Work out the finished part from the listing and answer in its coordinate system (mm). A direction names the side the tool comes from. Coordinates: 2 decimals unless noted, no trailing zeros. Loops run counter-clockwise (first coordinate to the right, second up) from the corner with the lowest first, then second, coordinate; pieces in that order, holes last.
Autodesk Inventor part; units mm, degrees
ref_plane "YZ Plane" through (0, 0, 0) normal (1, 0, 0) x (0, 1, 0)
ref_plane "XZ Plane" through (0, 0, 0) normal (0, 1, 0) x (-1, 0, 0)
ref_plane "XY Plane" through (0, 0, 0) normal (0, 0, 1) x (1, 0, 0)
sketch "Sketch1" plane through (0, 0, 0) normal (0, 1, 0) x (-1, 0, 0)
  line L0 (0, 0) -> (14.859, 0)
  line L1 (14.859, 0) -> (14.859, -17.145)
  line L2 (14.859, -17.145) -> (0, -17.145)
  line L3 (0, -17.145) -> (0, 0)
  line L4 (0, 0) -> (0, -1.143)
  line L5 (0, -1.143) -> (-3.175, -1.143)
  line L6 (-3.175, -1.143) -> (-20.32, -1.143)
  line L7 (-20.32, -1.143) -> (-20.32, -16.002)
  line L8 (-20.32, -16.002) -> (-3.175, -16.002)
  line L9 (-3.175, -16.002) -> (-3.175, -1.143)
  line L10 (14.859, 0) -> (14.859, 3.175)
  line L11 (14.859, 3.175) -> (18.034, 3.175)
  line L12 (-20.32, -1.143) -> (-23.495, -1.143)
  line L13 (-20.32, -16.002) -> (-20.32, -19.177)
  line L14 (-20.32, -19.177) -> (-23.495, -19.177)
  line L15 (18.034, 3.175) -> (-23.495, 3.175)
  line L16 (-23.495, 3.175) -> (-23.495, -19.177)
  line L17 (-23.495, -19.177) -> (18.034, -19.177)
  line L18 (18.034, -19.177) -> (18.034, 3.175)
  dimension "d0" = 14.859
  dimension "d1" = 17.145
  dimension "d2" = 1.143
  dimension "d3" = 3.175
  dimension "d4" = 17.145
  dimension "d5" = 14.859
  dimension "d6" = 3.175
  dimension "d7" = 3.175
  dimension "d8" = 3.175
  dimension "d34" = 3.175
  dimension "d35" = 3.175
extrude "Extrusion1" add sketch "Sketch1" along normal blind 25.4 contours L3 L5 L6 L12 L16 L15 L10 L0 | L10 L11 L18 L17 L13 L8 L9 L5 L3 L2 L1 | L7 L13 L14 L16 L12
sketch "Sketch2" plane through (23.495, 0, 1.5875) normal (1, 0, 0) x (0, 0, -1)
  line L0 (17.5895, 25.4) -> (2.7305, 25.4)
  line L1 (10.16, 25.4) -> (10.16, 17.399)
  circle A0 centre (10.16, 17.399) radius 1.5875
  line L2 (10.16, 17.399) -> (10.16, 2.413)
  circle A1 centre (10.16, 2.413) radius 1.5875
  point P0 (1.5875, 0)
  dimension "d13" = 8.001
  dimension "d14" = 3.175
  dimension "d15" = 14.986
  dimension "d16" = 3.175
extrude "Extrusion2" cut sketch "Sketch2" against normal blind 9.525
sketch "Sketch3" plane through (19.05, 0, -19.177) normal (0, 0, -1) x (-1, 0, 0)
  line L0 (33.909, 0) -> (33.909, 25.4)
  line L1 (19.05, 0) -> (19.05, 25.4)
  line L2 (33.909, 25.4) -> (19.05, 25.4)
  line L3 (26.4795, 25.4) -> (26.4795, 17.399)
  circle A0 centre (26.4795, 17.399) radius 1.5875
  line L4 (26.4795, 17.399) -> (26.4795, 2.413)
  circle A1 centre (26.4795, 2.413) radius 1.5875
  dimension "d19" = 8.001
  dimension "d20" = 3.175
  dimension "d21" = 14.986
  dimension "d22" = 3.175
extrude "Extrusion3" cut sketch "Sketch3" against normal blind 9.525
move faces "Move1" translate (0, -1.5875, 0) faces at (1.8203, 0, 2.1167)
sketch "Sketch4" plane through (-18.034, 25.4, -17.4625) normal (-1, 0, 0) x (0, 0, 1)
  line L0 (19.05, 0) -> (0, 0)
  line L1 (20.6375, -26.9875) -> (20.6375, 0)
  line L2 (-1.7145, -26.9875) -> (-1.7145, 0)
  line L3 (20.6375, 0) -> (-1.7145, 0)
  line L4 (-1.7145, 0) -> (-1.7145, -3.175)
  line L5 (-1.7145, -3.175) -> (20.6375, -3.175)
  line L6 (20.6375, -3.175) -> (20.6375, 0)
  point P0 (17.4625, -25.4)
  point P1 (20.6375, -3.175)
  dimension "d36" = 3.175
extrude "Extrusion4" add sketch "Sketch4" along normal blind 20.32
sketch "Sketch5" plane through (-15.1765, 25.4, -17.4625) normal (0, -1, 0) x (1, 0, 0)
  line L0 (-23.1775, 20.6375) -> (-23.1775, -1.7145)
  line L1 (0.3175, 17.4625) -> (0.3175, 0.3175)
  line L2 (-23.1775, 9.4615) -> (0.3175, 9.4615) construction
  line L3 (-23.1775, 9.4615) -> (-2.8575, 9.4615)
  line L4 (-2.8575, -1.7145) -> (-2.8575, 20.6375)
  circle A0 centre (-13.0175, 9.4615) radius 2.54
  point P0 (15.1765, 17.4625)
  dimension "d39" = 5.08
extrude "Extrusion5" cut sketch "Sketch5" along normal blind 14.605
properties part number "PluckMount"
1. A cutting plane is placed at D-D, the plane x = 5.5. Give the vertices of the cut face in (y, z) (1 decimal).
2. For faces 4 (the cylindrical face through (-6.259, 3.486, -18.175)), 5 (the flat face through (-18.034, 10, -8)), 6 (the cylindrical face through (21.93, 3.486, -7.402)), 7 (the flat face through (-7, 12, 0)), determine the directions among +Z, -Z, +X, -X, +Y, -Y from which every point of the face is accessible in a straight line to the end or side of a thin tool.
3. A cutting plane is placed at B-B, the plane z = -14.75. Give the vertices of the cut face in (x, y) (1 decimal).
4. A cutting plane is placed at A-A, the plane x = -11.5. Give the vertices of the cut face in (y, z) (1 decimal).
5. A cutting plane is placed at C-C, the plane y = 14.5. Give the vertices of the cut face in (x, z) (3 decimals).
6. Determine the mould class of faces 1 (the cylindrical face through (-6.26, 18.47, -18.18)), 2 (the flat face through (-14.859, 12, -8)), 3 (the flat face through (0, 12, -19.177)) for opening direction Z: released by +Z, released by -Z, zero draft, split by the parting line, or undercut.
7. Each of these flat-tipped pins is pushed along its axis until it touches: P1, Ø5, axis at x = -2, z = -1, coming from the +Y side; P2, Ø2.5, axis at y = 17.4, z = -8.57, coming from the -X side; P3, Ø1.9, axis at y = 2.41, z = -8.57, coming from the +X side (3 decimals). Where does it stop, or does it pass through?
8. Straight lines are drawn through the part: probe 1 along X at (y, z) = (15.25, -7.5) (3 decimals); probe 2 along Z at (x, y) = (9.5, 4) (3 decimals); probe 3 along X at (y, z) = (24, -13.75) (3 decimals). For each, find the intervals that lie inside material, in ascending order.
Answers below:
1. outline: (-1.6, -19.2) - (25.4, -19.2) - (25.4, -16) - (-1.6, -16) - close; (-1.6, -1.1) - (25.4, -1.1) - (25.4, 3.2) - (-1.6, 3.2) - close
2. face 4: -Z
2. face 5: +Z, -Z, -X, -Y
2. face 6: +X
2. face 7: +Y, -Y
3. outline: (-38.4, 22.2) - (-18, 22.2) - (-18, -1.6) - (-14.9, -1.6) - (-14.9, 25.4) - (-38.4, 25.4) - close; (0, -1.6) - (3.2, -1.6) - (3.2, 25.4) - (0, 25.4) - close; (20.3, -1.6) - (23.5, -1.6) - (23.5, 25.4) - (20.3, 25.4) - close
4. outline: (-1.6, -19.2) - (25.4, -19.2) - (25.4, -17.1) - (-1.6, -17.1) - close; (-1.6, 0) - (25.4, 0) - (25.4, 3.2) - (-1.6, 3.2) - close
5. outline: (-18.034, -19.177) - (23.495, -19.177) - (23.495, 3.175) - (-18.034, 3.175) - close; hole (-14.859, -17.145) - (0, -17.145) - (0, 0) - (-14.859, 0) - close; hole (3.175, -16.002) - (20.32, -16.002) - (20.32, -1.143) - (3.175, -1.143) - close
6. face 1: zero draft
6. face 2: undercut
6. face 3: released by -Z
7. P1: stops at y = 25.4
7. P2: stops at x = -18.03
7. P3: stops at x = 3.175
8. probe 1: x = -18.034 to -14.859, 0 to 3.175, 20.32 to 23.495
8. probe 2: z = -19.177 to -16.002, -1.143 to 3.175
8. probe 3: x = -38.354 to -14.859, 0 to 3.175, 20.32 to 23.495
